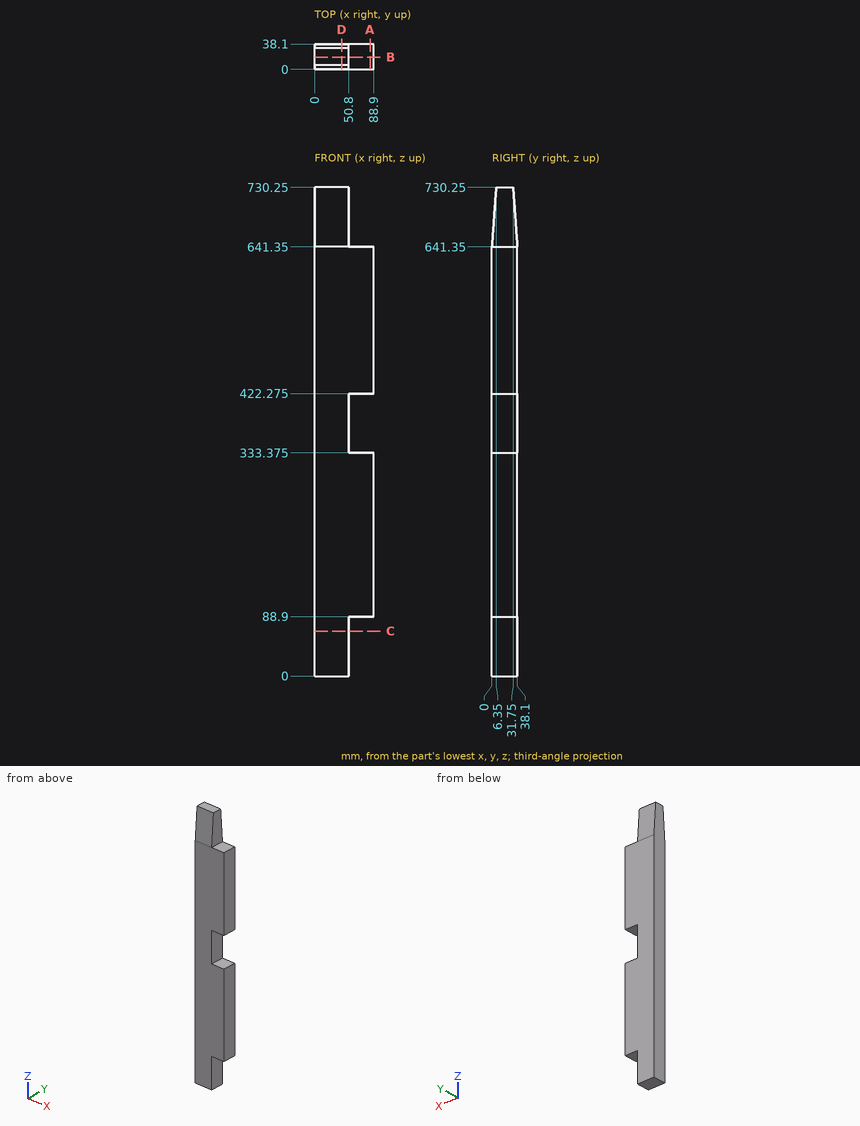
Answer from the drawing. Dimensions are ordinates in mm from the lowest x, y and z of the part. Coordinates: 2 decimals unless noted, no trailing zeros. Write each loop counter-clockwise with the first axis right and the second up, starting at its lowest first coordinate (ties: lowest second). Pieces come first, ordered by that corner, then holes. Notation, with made-up numbers: (-39, 44) - (-4, 44) arc R26 ccw to (-4, 66) - close; hole circle Ø8 at (35.5, 9). An arc over 180 degrees is marked (long way). Return JSON: item names as keys, results as strings. Group by question number.
Q1. The part is cut by section B-B on y = 18.5. Write down the section's boundary in (x, z) (3 decimals), and give its area (3 significant figures).
Q2. Flat-ended cylindrical pins translate along their axes: pin 1 Ø19 at (y, z) = (20.5, 65.5) entering from +X; pin 2 Ø11.5 at (x, y) = (70.5, 18) entering from +Z; pin 3 Ø4 at (x, y) = (72.5, 24.5) entering from -Z. Find the tip coordinate at first contact, or state that the pin passes through.
Q3. The part is cut by section C-C on z = 67. Write down the section's boundary in (x, y), and give its area (3 significant figures).
Q4. The part is cut by section D-D on x = 40.5. Write down the section's boundary in (y, z), and give its area (3 significant figures).
Q5. The part is cut by section A-A on x = 83. Write down the section's boundary in (y, z) (3 decimals), and give its area (3 significant figures).
Q6. Find the intervals of material crossed by line 1 along Z through (x, y) = (53, 25.5) (3 decimals); line 2 along X through (y, z) = (27, 370), in increasing order. Write a range as [from, to].
Evaluation:
{
 "1": {"outline": "(0, 0) - (50.8, 0) - (50.8, 88.9) - (88.9, 88.9) - (88.9, 333.375) - (50.8, 333.375) - (50.8, 422.275) - (88.9, 422.275) - (88.9, 641.35) - (50.8, 641.35) - (50.8, 730.25) - (0, 730.25) - close", "area": "54,800 mm2"},
 "2": {"pin 1": "stops at x = 50.8", "pin 2": "stops at z = 641.35", "pin 3": "stops at z = 88.9"},
 "3": {"outline": "(0, 0) - (50.8, 0) - (50.8, 38.1) - (0, 38.1) - close", "area": "1,940 mm2"},
 "4": {"outline": "(0, 0) - (38.1, 0) - (38.1, 641.35) - (31.75, 730.25) - (6.35, 730.25) - (0, 641.35) - close", "area": "27,300 mm2"},
 "5": {"outline": "(0, 88.9) - (38.1, 88.9) - (38.1, 333.375) - (0, 333.375) - close; (0, 422.275) - (38.1, 422.275) - (38.1, 641.35) - (0, 641.35) - close", "area": "17,700 mm2"},
 "6": {"line 1": "z = [88.9, 333.375], [422.275, 641.35]", "line 2": "x = [0, 50.8]"}
}
